Source: CAD feature listing. Evaluate the final solid. Frame: model axes, mm. Round coordinates to 2 decimals unless told otherwise and drop trailing zeros. Use a Markdown table: item, result. Add a question column.
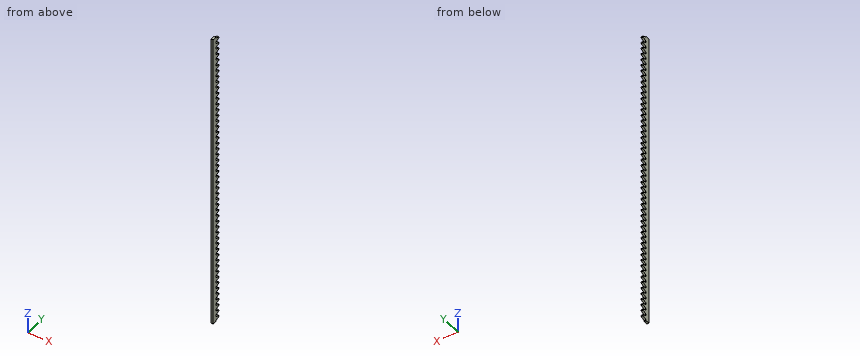
```python
from build123d import *

# Parameters (mm, degrees)
ESBO_O1_W                = 3
ESBO_O1_H                = 13
RESSALTO_EXTRUS_O1_DEPTH = 480.664
CORTE_EXTRUS_O1_DEPTH    = 481.849124878


with BuildPart() as part:
    # Esboço1 → Ressalto-extrusão1 (new body)
    with BuildSketch(Plane.XY):
        with Locations((1.5, 6.5)):
            Rectangle(ESBO_O1_W, ESBO_O1_H)
    extrude(amount=RESSALTO_EXTRUS_O1_DEPTH)

    # Esboço2 → Corte-extrusão1 (cut, through all)
    with BuildSketch(Plane.ZY):
        Polygon((1.312306109, 6.2246), (-1.312306109, 6.2246), (-3.778350034, 13), (3.778350034, 13), align=None)
        Polygon((10.737084059, 6.2246), (8.112471841, 6.2246), (5.646427916, 13), (13.203127984, 13), align=None)
        Polygon((20.161862009, 6.2246), (17.537249791, 6.2246), (15.071205866, 13), (22.627905934, 13), align=None)
        Polygon((29.586639959, 6.2246), (26.962027741, 6.2246), (24.495983816, 13), (32.052683884, 13), align=None)
        Polygon((39.011417909, 6.2246), (36.386805691, 6.2246), (33.920761766, 13), (41.477461834, 13), align=None)
        Polygon((48.436195859, 6.2246), (45.811583641, 6.2246), (43.345539716, 13), (50.902239784, 13), align=None)
        Polygon((57.860973809, 6.2246), (55.236361591, 6.2246), (52.770317666, 13), (60.327017734, 13), align=None)
        Polygon((67.285751759, 6.2246), (64.661139541, 6.2246), (62.195095616, 13), (69.751795684, 13), align=None)
        Polygon((76.710529709, 6.2246), (74.085917491, 6.2246), (71.619873566, 13), (79.176573634, 13), align=None)
        Polygon((86.135307659, 6.2246), (83.510695441, 6.2246), (81.044651516, 13), (88.601351584, 13), align=None)
        Polygon((95.560085609, 6.2246), (92.935473391, 6.2246), (90.469429466, 13), (98.026129534, 13), align=None)
        Polygon((104.984863559, 6.2246), (102.360251341, 6.2246), (99.894207416, 13), (107.450907484, 13), align=None)
        Polygon((114.409641509, 6.2246), (111.785029291, 6.2246), (109.318985366, 13), (116.875685434, 13), align=None)
        Polygon((123.834419459, 6.2246), (121.209807241, 6.2246), (118.743763316, 13), (126.300463384, 13), align=None)
        Polygon((133.259197409, 6.2246), (130.634585191, 6.2246), (128.168541266, 13), (135.725241334, 13), align=None)
        Polygon((142.683975359, 6.2246), (140.059363141, 6.2246), (137.593319216, 13), (145.150019284, 13), align=None)
        Polygon((152.108753309, 6.2246), (149.484141091, 6.2246), (147.018097166, 13), (154.574797234, 13), align=None)
        Polygon((161.533531259, 6.2246), (158.908919041, 6.2246), (156.442875116, 13), (163.999575184, 13), align=None)
        Polygon((170.958309209, 6.2246), (168.333696991, 6.2246), (165.867653066, 13), (173.424353134, 13), align=None)
        Polygon((180.383087159, 6.2246), (177.758474941, 6.2246), (175.292431016, 13), (182.849131084, 13), align=None)
        Polygon((189.807865109, 6.2246), (187.183252891, 6.2246), (184.717208966, 13), (192.273909034, 13), align=None)
        Polygon((199.232643059, 6.2246), (196.608030841, 6.2246), (194.141986916, 13), (201.698686984, 13), align=None)
        Polygon((208.657421009, 6.2246), (206.032808791, 6.2246), (203.566764866, 13), (211.123464934, 13), align=None)
        Polygon((218.082198959, 6.2246), (215.457586741, 6.2246), (212.991542816, 13), (220.548242884, 13), align=None)
        Polygon((227.506976909, 6.2246), (224.882364691, 6.2246), (222.416320766, 13), (229.973020834, 13), align=None)
        Polygon((236.931754859, 6.2246), (234.307142641, 6.2246), (231.841098716, 13), (239.397798784, 13), align=None)
        Polygon((246.356532809, 6.2246), (243.731920591, 6.2246), (241.265876666, 13), (248.822576734, 13), align=None)
        Polygon((255.781310759, 6.2246), (253.156698541, 6.2246), (250.690654616, 13), (258.247354684, 13), align=None)
        Polygon((265.206088709, 6.2246), (262.581476491, 6.2246), (260.115432566, 13), (267.672132634, 13), align=None)
        Polygon((274.630866659, 6.2246), (272.006254441, 6.2246), (269.540210516, 13), (277.096910584, 13), align=None)
        Polygon((284.055644609, 6.2246), (281.431032391, 6.2246), (278.964988466, 13), (286.521688534, 13), align=None)
        Polygon((293.480422559, 6.2246), (290.855810341, 6.2246), (288.389766416, 13), (295.946466484, 13), align=None)
        Polygon((302.905200509, 6.2246), (300.280588291, 6.2246), (297.814544366, 13), (305.371244434, 13), align=None)
        Polygon((312.329978459, 6.2246), (309.705366241, 6.2246), (307.239322316, 13), (314.796022384, 13), align=None)
        Polygon((321.754756409, 6.2246), (319.130144191, 6.2246), (316.664100266, 13), (324.220800334, 13), align=None)
        Polygon((331.179534359, 6.2246), (328.554922141, 6.2246), (326.088878216, 13), (333.645578284, 13), align=None)
        Polygon((340.604312309, 6.2246), (337.979700091, 6.2246), (335.513656166, 13), (343.070356234, 13), align=None)
        Polygon((350.029090259, 6.2246), (347.404478041, 6.2246), (344.938434116, 13), (352.495134184, 13), align=None)
        Polygon((359.453868209, 6.2246), (356.829255991, 6.2246), (354.363212066, 13), (361.919912134, 13), align=None)
        Polygon((368.878646159, 6.2246), (366.254033941, 6.2246), (363.787990016, 13), (371.344690084, 13), align=None)
        Polygon((378.303424109, 6.2246), (375.678811891, 6.2246), (373.212767966, 13), (380.769468034, 13), align=None)
        Polygon((387.728202059, 6.2246), (385.103589841, 6.2246), (382.637545916, 13), (390.194245984, 13), align=None)
        Polygon((397.152980009, 6.2246), (394.528367791, 6.2246), (392.062323866, 13), (399.619023934, 13), align=None)
        Polygon((406.577757959, 6.2246), (403.953145741, 6.2246), (401.487101816, 13), (409.043801884, 13), align=None)
        Polygon((416.002535909, 6.2246), (413.377923691, 6.2246), (410.911879766, 13), (418.468579834, 13), align=None)
        Polygon((425.427313859, 6.2246), (422.802701641, 6.2246), (420.336657716, 13), (427.893357784, 13), align=None)
        Polygon((434.852091809, 6.2246), (432.227479591, 6.2246), (429.761435666, 13), (437.318135734, 13), align=None)
        Polygon((444.276869759, 6.2246), (441.652257541, 6.2246), (439.186213616, 13), (446.742913684, 13), align=None)
        Polygon((453.701647709, 6.2246), (451.077035491, 6.2246), (448.610991566, 13), (456.167691634, 13), align=None)
        Polygon((463.126425659, 6.2246), (460.501813441, 6.2246), (458.035769516, 13), (465.592469584, 13), align=None)
        Polygon((472.551203609, 6.2246), (469.926591391, 6.2246), (467.460547466, 13), (475.017247534, 13), align=None)
        Polygon((481.975981559, 6.2246), (479.351369341, 6.2246), (476.885325416, 13), (484.442025484, 13), align=None)
    extrude(amount=-CORTE_EXTRUS_O1_DEPTH, mode=Mode.SUBTRACT)


solid = part.part
```
1) Section A-A on y = 9.75. Count the separate pieces of the cut face and the enclosed holes in it, then the cut area to 3 significant figures.
2) First-contact query: pin 1 Ø0.8 at (x, z) = (2, 245.5) entering from +Y. Flat tip, straight axial feed; report the tip coordinate or a pass-through.
3) Line query: probe 1 along Y at (x, z) = (2.8, 85). Output: solid intervals per line, ascending. Write a range as from..to.
Conclusion:
| question | item | result |
|---|---|---|
| 1 | separate pieces | 51 |
| 1 | enclosed holes | 0 |
| 1 | area | 648 mm^2 |
| 2 | pin 1 | stops at y = 6.22 |
| 3 | probe 1 | y = 0..6.22 |
